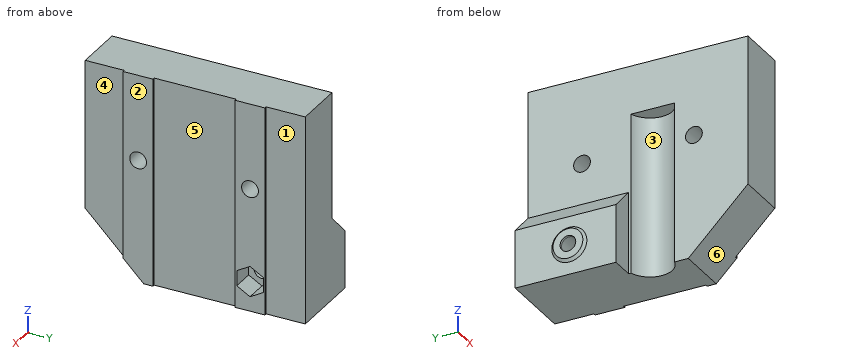
```python
from build123d import *

# Parameters (mm, degrees)
BOSS_EXTRUDE1_DEPTH                          = 10
BOSS_EXTRUDE1_2_DEPTH                        = 10
CBORE_FOR_M5_HEX_SOCKET_HEAD_CAP_SCR_2_COUNT = 2
CBORE_FOR_M5_HEX_SOCKET_HEAD_CAP_SCR_2_PITCH = 30
BOSS_EXTRUDE2_DEPTH                          = 13
BOSS_EXTRUDE3_DEPTH                          = 23
BOSS_EXTRUDE4_DEPTH                          = 27
SKETCH8_R                                    = 2.1
CUT_EXTRUDE1_DEPTH                           = 52.298148115
CHAMFER1_SIZE                                = 16
CUT_EXTRUDE2_DEPTH                           = 6
SKETCH10_R                                   = 5
SKETCH10_R_2                                 = 2.1
BOSS_EXTRUDE5_DEPTH                          = 0.7
CHAMFER2_SIZE                                = 1


with BuildPart() as part:
    # Sketch1 → Boss-Extrude1 (new, symmetric)
    with BuildSketch(Plane.XY):
        with BuildLine():
            Line((-14, 32.5), (-1.5, 32.5))
            Line((-1.5, 32.5), (-1.5, 5.809475019))
            ThreePointArc((-1.5, 5.809475019), (-6, 0), (-1.5, -5.809475019))
            Line((-1.5, -5.809475019), (-1.5, -24.5))
            Line((-1.5, -24.5), (-14, -24.5))
            Line((-14, -24.5), (-14, 32.5))
        make_face()
    extrude(amount=BOSS_EXTRUDE1_DEPTH, both=True)


with BuildPart() as body_2:
    # Sketch1 → Boss-Extrude1 2 (new, symmetric)
    with BuildSketch(Plane.XY):
        with BuildLine():
            Line((15, 33.5), (15, 23))
            Line((15, 23), (15.6, 23))
            Line((15.6, 23), (15.6, 15))
            Line((15.6, 15), (15, 15))
            Line((15, 15), (15, -7))
            Line((15, -7), (15.6, -7))
            Line((15.6, -7), (15.6, -15))
            Line((15.6, -15), (15, -15))
            Line((15, -15), (15, -25.5))
            Line((15, -25.5), (1.5, -25.5))
            Line((1.5, -25.5), (1.5, -5.809475019))
            ThreePointArc((1.5, -5.809475019), (6, 0), (1.5, 5.809475019))
            Line((1.5, 5.809475019), (1.5, 33.5))
            Line((1.5, 33.5), (15, 33.5))
        make_face()
    extrude(amount=BOSS_EXTRUDE1_2_DEPTH, both=True)


with BuildPart() as cbore_for_m5_hex_socket_head_cap_screw1_tool:
    # Sketch2 → CBORE for M5 Hex Socket Head Cap Screw1 (revolve)
    with BuildSketch(Plane(origin=(-14, -11, 0), x_dir=(0, 0, 1), z_dir=(0, 1, 0))):
        Polygon((0, 0), (0, 29.6), (2.25, 29.6), (2.25, 5.9), (5, 5.9), (5, 0), align=None)
    cbore_for_m5_hex_socket_head_cap_screw1 = revolve(axis=Axis((-20.35, -11, 0), (1, 0, 0)))


with BuildPart() as part_1:
    add(part.part)

    # CBORE for M5 Hex Socket Head Cap Screw1: cut by cbore_for_m5_hex_socket_head_cap_screw1_tool
    add(cbore_for_m5_hex_socket_head_cap_screw1_tool.part, mode=Mode.SUBTRACT)


with BuildPart() as body_2_1:
    add(body_2.part)

    # CBORE for M5 Hex Socket Head Cap Screw1: cut by cbore_for_m5_hex_socket_head_cap_screw1_tool
    add(cbore_for_m5_hex_socket_head_cap_screw1_tool.part, mode=Mode.SUBTRACT)


with BuildPart() as cbore_for_m5_hex_socket_head_cap_scr_2_tool:
    # CBORE for M5 Hex Socket Head Cap Scr 2: CBORE for M5 Hex Socket Head Cap Screw1 ×2
    with Locations(*[(0, i * CBORE_FOR_M5_HEX_SOCKET_HEAD_CAP_SCR_2_PITCH, 0) for i in range(1, CBORE_FOR_M5_HEX_SOCKET_HEAD_CAP_SCR_2_COUNT)]):
        add(cbore_for_m5_hex_socket_head_cap_screw1)


with BuildPart() as part_2:
    add(part_1.part)

    # CBORE for M5 Hex Socket Head Cap Scr 2: cut by cbore_for_m5_hex_socket_head_cap_scr_2_tool
    add(cbore_for_m5_hex_socket_head_cap_scr_2_tool.part, mode=Mode.SUBTRACT)


with BuildPart() as body_2_2:
    add(body_2_1.part)

    # CBORE for M5 Hex Socket Head Cap Scr 2: cut by cbore_for_m5_hex_socket_head_cap_scr_2_tool
    add(cbore_for_m5_hex_socket_head_cap_scr_2_tool.part, mode=Mode.SUBTRACT)

    # Sketch4 → Boss-Extrude2 (add)
    with BuildSketch(Plane.XY.offset(10)):
        Polygon((1.5, 5.809475019), (1.5, -5.809475019), (1.5, -25.5), (15, -25.5), (15, -15), (15.6, -15), (15.6, -7), (15, -7), (15, 15), (15.6, 15), (15.6, 23), (15, 23), (15, 33.5), (1.5, 33.5), align=None)
    extrude(amount=BOSS_EXTRUDE2_DEPTH)

    # Sketch5 → Boss-Extrude3 (add)
    with BuildSketch(Plane(origin=(0, 0, -10), x_dir=(-1, 0, 0), z_dir=(0, 0, -1))):
        with BuildLine():
            Line((-15, -25.5), (-1.5, -25.5))
            Line((-1.5, -25.5), (-1.5, -5.809475019))
            ThreePointArc((-1.5, -5.809475019), (-6, 0), (-1.5, 5.809475019))
            Line((-1.5, 5.809475019), (-1.5, 33.5))
            Line((-1.5, 33.5), (-15, 33.5))
            Line((-15, 33.5), (-15, 23))
            Line((-15, 23), (-15.6, 23))
            Line((-15.6, 23), (-15.6, 15))
            Line((-15.6, 15), (-15, 15))
            Line((-15, 15), (-15, -7))
            Line((-15, -7), (-15.6, -7))
            Line((-15.6, -7), (-15.6, -15))
            Line((-15.6, -15), (-15, -15))
            Line((-15, -15), (-15, -25.5))
        make_face()
    extrude(amount=BOSS_EXTRUDE3_DEPTH)

    # Sketch7 → Boss-Extrude4 (add)
    with BuildSketch(Plane(origin=(0, 33.5, 0), x_dir=(1, 0, 0), z_dir=(0, 1, 0))):
        Polygon((1.5, 33), (-4.9, 33), (-4.9, 17.4), (1.5, 11), align=None)
    extrude(amount=-BOSS_EXTRUDE4_DEPTH)

    # Sketch8 → Cut-Extrude1 (cut, through all)
    with BuildSketch(Plane.ZY.offset(4.9)):
        with Locations((-25, 19)):
            Circle(SKETCH8_R)
    extrude(amount=-CUT_EXTRUDE1_DEPTH, mode=Mode.SUBTRACT)

    # Chamfer1
    chamfer1_edges = [body_2_2.edges().sort_by_distance(p)[0] for p in [
        (8.25, -25.5, -33),
    ]]
    chamfer(chamfer1_edges, length=CHAMFER1_SIZE)

    # Sketch9 → Cut-Extrude2 (cut)
    with BuildSketch(Plane(origin=(15.6, 0, 0), x_dir=(0, 0, -1), z_dir=(1, 0, 0))):
        Polygon((29.099186911, 19), (27.049593456, 22.55), (22.950406544, 22.55), (20.900813089, 19), (22.950406544, 15.45), (27.049593456, 15.45), align=None)
    extrude(amount=-CUT_EXTRUDE2_DEPTH, mode=Mode.SUBTRACT)

    # Sketch10 → Boss-Extrude5 (add)
    with BuildSketch(Plane.ZY.offset(4.9)):
        with Locations((-25, 19)):
            Circle(SKETCH10_R)
        with Locations((-25, 19)):
            Circle(SKETCH10_R_2, mode=Mode.SUBTRACT)
    extrude(amount=BOSS_EXTRUDE5_DEPTH)

    # Chamfer2
    # the kernel refuses this chamfer: 1 mm, written as the material it takes off along each edge
    with BuildSketch(Plane(origin=(-5.6, 19, -25), x_dir=(0, 0, 1), z_dir=(0, -1, 0))) as chamfer2_piece_1_section:
        Polygon((5, -CHAMFER2_SIZE), (5 - CHAMFER2_SIZE, 0), (5, 0), align=None)
    chamfer2_piece_1 = revolve(axis=Axis((-5.6, 19, -25), (-1, 0, 0)), mode=Mode.PRIVATE)
    chamfer2_piece_1 = split(chamfer2_piece_1, bisect_by=Plane(origin=(-4.9, 19, -29.353058273), z_dir=(-1, 0, 0)), keep=Keep.TOP, mode=Mode.PRIVATE)
    add(chamfer2_piece_1, mode=Mode.SUBTRACT)


solid = body_2_2.part
```
Geometry check sheet. Reference: the model listing, model coordinates, mm. Face numbers are marked on the shaded views. A direction names the side the tool comes from. Coordinates: 2 decimals unless noted, no trailing zeros. Loops run counter-clockwise (first coordinate to the right, second up) from the corner with the lowest first, then second, coordinate; pieces in that order, holes last. Notation, with made-up numbers: (-16.75, 71.25) - (31.25, 71.25) arc R31 cw to (31.25, 100.25) - close; hole circle Ø7 at (1, 82.5). An arc over 180 degrees is marked (long way). One line per item, written item: value. Start each with the question number.
(1) Cross-section at A-A on z = 0. Enter the section's corners in (x, y), plus the area to 3 significant figures.
(2) Cross-section at C-C on y = -11. Enter the section's corners in (x, z).
(3) Cross-section at D-D on z = -25. Enter the section's corners in (x, y).
(4) Depth check by flat-ended pin: P1, Ø1.2, axis at x = 13.5, z = -24.5, coming from the -Y side; P2, Ø3, axis at x = -1, z = -23, coming from the -Y side; P3, Ø6, axis at y = -11, z = 0, coming from the -X side. Enter the tip coordinate at first touch or a pass-through.
(5) Material ranges on line 1 (Y direction, x = 14, z = 0); line 2 (Y direction, x = 5.25, z = 0); line 3 (Y direction, x = 5.5, z = 0), recorded low to high. Write a range as [from, to].
(6) Cross-section at B-B on x = 13.75. Enter the section's corners in (y, z).
(7) Tool access check on the marked faces 1, 2 and 3. Record the directions out of +Z, -Z, +X, -X, +Y, -Y that give a thin tool (end or side, any length) a straight path to the whole face; none if there is none.
(8) Mould release check, pull along Y, two halves, no side actions. Record for the marked faces 4, 5 and 6: released by +Y, released by -Y, zero draft, split by the parting line, or undercut.
Results below:
1. outline: (1.5, -25.5) - (15, -25.5) - (15, -15) - (15.6, -15) - (15.6, -13.25) - (1.5, -13.25) - close; (1.5, -8.75) - (15.6, -8.75) - (15.6, -7) - (15, -7) - (15, 15) - (15.6, 15) - (15.6, 16.75) - (1.5, 16.75) - (1.5, 5.81) arc R6 cw to (1.5, -5.81) - close; (1.5, 21.25) - (15.6, 21.25) - (15.6, 23) - (15, 23) - (15, 33.5) - (1.5, 33.5) - close
1. area: 640 mm2
2. outline: (1.5, -31.5) - (15.6, -31.5) - (15.6, -2.25) - (1.5, -2.25) - close; (1.5, 2.25) - (15.6, 2.25) - (15.6, 23) - (1.5, 23) - close
3. outline: (-5.6, 15) - (-4.9, 14.3) - (-4.9, 6.5) - (1.5, 6.5) - (1.5, 5.81) arc R6 cw to (1.5, -5.81) - (1.5, -17.5) - (15, -17.5) - (15, -15) - (15.6, -15) - (15.6, -7) - (15, -7) - (15, 15) - (15.6, 15) - (15.6, 15.45) - (9.6, 15.45) - (9.6, 16.9) - (-5.6, 16.9) - close; (-5.6, 21.1) - (9.6, 21.1) - (9.6, 22.55) - (15.6, 22.55) - (15.6, 23) - (15, 23) - (15, 33.5) - (-4.9, 33.5) - (-4.9, 23.7) - (-5.6, 23) - close
4. P1: stops at y = -18.6
4. P2: stops at y = 6.5
4. P3: stops at x = 1.5
5. line 1: y = [-25.5, -13.25], [-8.75, 16.75], [21.25, 33.5]
5. line 2: y = [-25.5, -13.25], [-8.75, -2.9], [2.9, 16.75], [21.25, 33.5]
5. line 3: y = [-25.5, -13.25], [-8.75, -2.4], [2.4, 16.75], [21.25, 33.5]
6. outline: (-25.5, -17) - (-9.5, -33) - (33.5, -33) - (33.5, 23) - (-25.5, 23) - close; hole circle Ø4.5 at (-11, 0); hole (15.45, -27.05) - (19, -29.1) - (22.55, -27.05) - (22.55, -22.95) - (19, -20.9) - (15.45, -22.95) - close; hole circle Ø4.5 at (19, 0)
7. face 1: +Z, -Z, +X, +Y
7. face 2: +Z, -Z, +X, +Y, -Y
7. face 3: -Z, -X
8. face 4: zero draft
8. face 5: undercut
8. face 6: released by -Y
